Autodesk Inventor part; units mm, degrees
ref_plane "Konstruktionshilfsebene" through (0, 4, 0) normal (0, 1, 0) x (-1, 0, 0)
ref_plane "YZ Plane" through (0, 0, 0) normal (1, 0, 0) x (0, 1, 0)
ref_plane "XY Plane" through (0, 0, 0) normal (0, 0, 1) x (1, 0, 0)
sketch "Skizze1" plane through (0, 0, 0) normal (0, 0, 1) x (1, 0, 0)
  arc A0 (0, 4) -> (0, -4) centre (0, 0) ccw
  line L0 (0, 4) -> (0, -4)
  line L1 (0, -5.6) -> (0, 5.6) construction
  dimension "d0" = 8
revolve "Kugelkörper" add sketch "Skizze1" angle 360 about axis through (0, -10, 0) along (0, 1, 0)
ref_plane "Konstruktionshilfsebene" through (0, 4, 0) normal (0, 1, 0) x (-1, 0, 0)
sketch "Skizze2" plane through (0, 4, 0) normal (0, 1, 0) x (-1, 0, 0)
  circle A0 centre (0, 0) radius 2.5
  point P0 (0, 0)
  dimension "d2" = 5
extrude "Gewindeschraube" add sketch "Skizze2" against normal blind 1 and the other way blind 15
chamfer "Gewindefase M3" distance 0.8 angle 45 1 edges at (2.5, 19, 0)
ref_plane "Work Plane2" through (0, 8.2, 0) normal (0, 1, 0) x (1, 0, 0)
sketch "Sketch3" plane through (0, 8.2, 0) normal (0, 1, 0) x (1, 0, 0)
  circle A0 centre (0, 0) radius 4
  line L0 (-1.9365, -3.5) -> (1.9365, -3.5)
  line L1 (-1.9365, 3.5) -> (1.9365, 3.5)
  dimension "d13" = 8
  dimension "d14" = 7
extrude "Extrusion2" add sketch "Sketch3" against normal blind 2.5 contours A0 L0 L1
thread "Thread2"
properties part number "Ball_Joint_Ball" material "Stahl, galvanisiert"
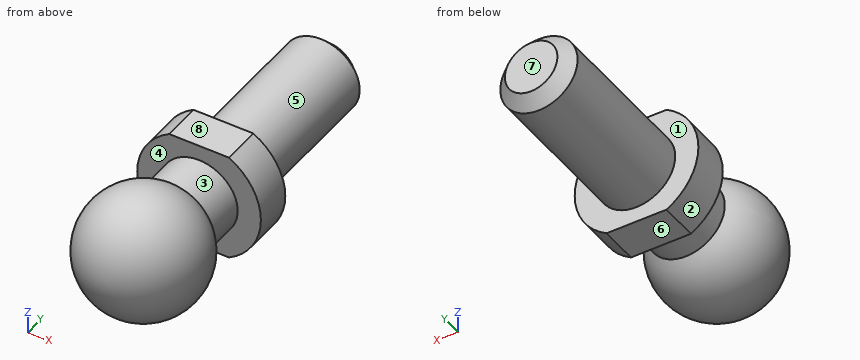
Check sheet for the modelled part. Datum: model origin and axes. Units: mm. Face numbers are marked on the shaded views. A direction names the side the tool comes from. Give positions to 0.01 mm unless a question says otherwise; leave off trailing zeros. Order: outer loops, then holes, each group sorted by start corner. A loop starts at its lowest first (then second) coordinate and runs counter-clockwise, first axis right, second up. Notation, with made-up numbers: M 4,79.5 L 38,79.5 A21 ccw 38,101.5 Z; hole C -21,81 d3. An arc over 180 degrees is marked long. Answer as CSV lines item,"result". Start each with the question number.
Item 1: Thickness scan on line 1 (Y direction, x = -2, z = 2.25); line 2 (Y direction, x = 3, z = -1.5); line 3 (Z direction, x = -3.5, y = 6). Record the ranges inside material, lowest first. Write a range as [from, to].
Item 2: Cross-section at B-B on x = 0. Enter the section's corners in (y, z).
Item 3: Cross-section at C-C on x = 2.75. Enter the section's corners in (y, z), plus the area to 3 significant figures.
Item 4: Tool access check on the marked faces 4, 5, 6, 7 and 8. Record the directions out of +Z, -Z, +X, -X, +Y, -Y that give a thin tool (end or side, any length) a straight path to the whole face; none if there is none.
Item 5: Cross-section at A-A on z = 0. Enter the section's corners in (x, y), plus the area to 3 significant figures.
Item 6: Cross-section at D-D on y = 16.5. Enter the section's corners in (x, z).
Item 7: Mould release check, pull along Y, two halves, no side actions. Record for the marked faces 1, 2 and 3: +Y half, -Y half, draft (parallel to the pull), parting line (faces both ways), or undercut.
Item 8: Gauge pin test, flat ends, axial feed: P1, Ø3, axis at y = -0.5, z = -3, coming from the -X side; P2, Ø2, axis at x = 0, y = 7, coming from the +Z side; P3, Ø1.2, axis at x = 0, y = 7.5, coming from the -Z side. Record the tip position at first contact, or that the pin passes through.
Established:
1,line 1,"y = [-2.63, 2.63], [5.7, 8.2]"
1,line 2,"y = [-2.18, 2.18], [5.7, 8.2]"
1,line 3,"z = [-1.94, 1.94]"
2,outline,"M 3.12,-2.5 L 5.7,-2.5 L 5.7,-3.5 L 8.2,-3.5 L 8.2,-2.5 L 18.2,-2.5 L 19,-1.7 L 19,1.7 L 18.2,2.5 L 8.2,2.5 L 8.2,3.5 L 5.7,3.5 L 5.7,2.5 L 3.12,2.5 A4 ccw long Z"
3,outline,"C 0,0 d5.81; M 5.7,-2.9 L 8.2,-2.9 L 8.2,2.9 L 5.7,2.9 Z"
3,area,"41.0 mm^2"
4,face 4,"none"
4,face 5,"+Y"
4,face 6,"-Z, +X, -X, +Y"
4,face 7,"+Z, -Z, +X, -X, +Y"
4,face 8,"+Z, +X, -X, +Y"
5,outline,"M -4,5.7 L -2.5,5.7 L -2.5,3.12 A4 ccw long 2.5,3.12 L 2.5,5.7 L 4,5.7 L 4,8.2 L 2.5,8.2 L 2.5,18.2 L 1.7,19 L -1.7,19 L -2.5,18.2 L -2.5,8.2 L -4,8.2 Z"
5,area,"134 mm^2"
6,outline,"C 0,0 d5"
7,face 1,"+Y half"
7,face 2,"draft"
7,face 3,"undercut"
8,P1,"stops at x = -3.69"
8,P2,"stops at z = 3.5"
8,P3,"stops at z = -3.5"
